from build123d import *

# Parameters (mm, degrees)
SKETCH1_R        = 17.8054
BASEPULLEY_DEPTH = 20.32
GROOVE_DEPTH     = 10.16
GROOVES_COUNT    = 12
GROOVES_ANGLE    = 330
SKETCH4_W        = 5.08
SKETCH4_H        = 12.7
BORSKE_R         = 4.7625
BORE_DEPTH       = 39.633634572


with BuildPart() as part:
    # Sketch1 → BasePulley (new body)
    with BuildSketch(Plane.XY):
        Circle(SKETCH1_R)
    extrude(amount=-BASEPULLEY_DEPTH)

    # Sketch2 → Flange (revolve)
    with BuildSketch(Plane(origin=(0, 0, 0), x_dir=(0, 0, -1), z_dir=(1, 0, 0)), mode=Mode.PRIVATE) as flange_sk:
        Polygon((20.32, 17.8054), (20.824761355, 19.4564), (22.039268395, 19.085087935), (21.59, 17.615597228), (21.59, 0), (-1.27, 0), (-1.27, 17.615597228), (-1.719268395, 19.085087935), (-0.504761355, 19.4564), (0, 17.8054), align=None)
    revolve(flange_sk.sketch.rotate(Axis((0, 0, 0), (0, 0, -1)), 90), axis=Axis((0, 0, 0), (0, 0, -1)))

    # Sketch3 → Groove (cut, symmetric)
    with BuildSketch(Plane.XY.offset(-10.16)):
        with BuildLine():
            Line((-2.3241, 17.8054), (-2.3241, 43.2054))
            Line((-2.3241, 43.2054), (2.3241, 43.2054))
            Line((2.3241, 43.2054), (2.3241, 17.8054))
            Line((2.3241, 17.8054), (1.752395126, 16.234653767))
            ThreePointArc((1.752395126, 16.234653767), (1.566408104, 15.992270762), (1.275031274, 15.9004))
            Line((1.275031274, 15.9004), (-1.275031274, 15.9004))
            ThreePointArc((-1.275031274, 15.9004), (-1.566408104, 15.992270762), (-1.752395126, 16.234653767))
            Line((-1.752395126, 16.234653767), (-2.3241, 17.8054))
        make_face()
    groove = extrude(amount=GROOVE_DEPTH, both=True, mode=Mode.SUBTRACT)

    # Grooves: Groove ×12 about axis
    grooves_axis = Axis((0, 0, -20.32), (0, 0, 1))
    for i in range(1, GROOVES_COUNT):
        add(groove.rotate(grooves_axis, i * GROOVES_ANGLE / (GROOVES_COUNT - 1)), mode=Mode.SUBTRACT)

    # Sketch4 → BaseHub (revolve)
    with BuildSketch(Plane(origin=(0, 0, 0), x_dir=(0, 0, -1), z_dir=(1, 0, 0)), mode=Mode.PRIVATE) as basehub_sk:
        with Locations((-2.54, 6.35)):
            Rectangle(SKETCH4_W, SKETCH4_H)
    revolve(basehub_sk.sketch.rotate(Axis((0, 0, 0), (0, 0, -1)), 277.328312747), axis=Axis((0, 0, 0), (0, 0, -1)))

    # BorSke → Bore (cut, through all)
    with BuildSketch(Plane.XY.offset(5.08)):
        Circle(BORSKE_R)
    extrude(amount=-BORE_DEPTH, mode=Mode.SUBTRACT)


solid = part.part
Read the model definition and answer for the solid it produces. Units are mm, in the model's axes. A direction names the side the tool comes from. Coordinates: 2 decimals unless noted, no trailing zeros. Write each loop counter-clockwise with the first axis right and the second up, starting at its lowest first coordinate (ties: lowest second). Pieces come first, ordered by that corner, then holes. Notation, with made-up numbers: (-35.75, -8) - (-13.75, -8) arc R8 ccw to (-13.75, 3) - close; hole circle Ø8 at (86.25, -15.5). An arc over 180 degrees is marked (long way). One line per question, with ' | ' between items.
Q1. For faces 1 (the flat face through (16.957, -2.015, -10.018)), 2 (the cylindrical face through (12.57, -12.61, -10.02)), 3 (the cylindrical face through (-4.6, -17.2, -10)), determine the directions among +Z, -Z, +X, -X, +Y, -Y from which every point of the face is accessible in a straight line to the end or side of a thin tool.
Result set:
face 1: +X | face 2: +X, -Y | face 3: -X, -Y
Q2. Consider L1, parallel to Y at x = 0, z = -6.75; L2, parallel to Z at x = 2, y = -14.5; L3, parallel to Z at x = 16.5, y = 1.5. Determine where each line is inside the solid, lowest interval first. Write a range as [from, to].
Result set:
L1: [-15.9, -4.76], [4.76, 15.9] | L2: [-21.59, 1.27] | L3: [-21.59, -20.32], [0, 1.27]
Q3. Find section A-A, the plane x = 0. Write down the section's boundary in (y, z).
Result set:
outline: (-19.46, -20.82) - (-19.09, -22.04) - (-17.62, -21.59) - (-4.76, -21.59) - (-4.76, 5.08) - (-12.7, 5.08) - (-12.7, 1.27) - (-17.62, 1.27) - (-19.09, 1.72) - (-19.46, 0.5) - (-17.81, 0) - (-15.9, 0) - (-15.9, -20.32) - (-17.81, -20.32) - close; (4.76, -21.59) - (17.62, -21.59) - (19.09, -22.04) - (19.46, -20.82) - (17.81, -20.32) - (15.9, -20.32) - (15.9, 0) - (17.81, 0) - (19.46, 0.5) - (19.09, 1.72) - (17.62, 1.27) - (12.7, 1.27) - (12.7, 5.08) - (4.76, 5.08) - close
Q4. Each of these flat-tipped pins is pushed along its axis until it touches: P1, Ø8, axis at x = 0.5, y = 4, coming from the -Z side; P2, Ø1, axis at x = 15.5, y = -8.5, coming from the +Z side; P3, Ø1, axis at x = 2.5, z = -2, coming from the -Y side. Where does it stop, or does it pass through?
Result set:
P1: z = -21.59 | P2: z = 1.44 | P3: y = -17.66
